Check sheet for the modelled part. Datum: model origin and axes. Units: mm. A direction names the side the tool comes from. Coordinates: 2 decimals unless noted, no trailing zeros. Loops run counter-clockwise (first coordinate to the right, second up) from the corner with the lowest first, then second, coordinate; pieces in that order, holes last. Notation, with made-up numbers: (84.5, 74) - (127.5, 74) arc R26 cw to (127.5, 91) - close; hole circle Ø11 at (3.25, -8.5). An arc over 180 degrees is marked (long way). Write each question's results on one line, items separated by ' | '. Start each with the question number.
1. Cross-section at C-C (y = -9). Record the cut outline in (x, z).
2. Thickness scan on line 1 (X direction, y = -5.5, z = 2.25); line 2 (X direction, y = 11, z = 1.5); line 3 (X direction, y = -10.5, z = 2). Record the ranges inside material, lowest first. Write a range as [from, to].
3. Draft check along X on faces 5 (the face through (40.14, 0.28, 5.9)), 6 (the face through (43, 0, 17)), 7 (the face through (17.5, -13, 2)). Enter one of: released by +X, released by -X, zero draft, split by the parting line, or undercut.
4. Gauge pin test, flat ends, axial feed: P1, Ø2.5, axis at y = -15.5, z = 3, coming from the -X side; P2, Ø2.5, axis at y = 5.5, z = 13, coming from the -X side; P3, Ø1.5, axis at x = -16, z = 3, coming from the -Y side; P4, Ø1.5, axis at y = 13.5, z = 1.5, coming from the -X side. Record the tip position at first contact, or that the pin passes through.
5. Cross-section at D-D (y = -16). Record the cut outline in (x, z), and give its area (3 significant figures).
6. Cross-section at A-A (z = 12). Record the cut outline in (x, y), and give its area (3 significant figures).
7. Cross-section at B-B (y = 4). Record the cut outline in (x, z), and give its area (3 significant figures).
8. Tool access check on faces 1 (the face through (27, -5.91, 2)), 2 (the face through (36, 15, 2)), 3 (the face through (43.465, 13.376, 12.066)), 4 (the face through (41, 0, 12)). Record the directions out of +Z, -Z, +X, -X, +Y, -Y that give a thin tool (end or side, any length) a straight path to the whole face; none if there is none.
```python
from build123d import *

# Parameters (mm, degrees)
F1_DEPTH = 5
F2_W     = 5
F2_H     = 40
F3_DEPTH = 12
F4_R     = 3
F5_R     = 1.5
F6_DEPTH = 10


with BuildPart() as f1:
    # F0 (on Top) → F1 (new body)
    with BuildSketch(Plane.XY):
        with BuildLine():
            Line((36, 18), (36, 10.910335))
            ThreePointArc((36, 10.910335), (34.535534, 7.374801), (31, 5.910335))
            Line((31, 5.910335), (19.677769, 5.910335))
            ThreePointArc((19.677769, 5.910335), (17.140309, 6.602052), (15.304931, 8.485816))
            ThreePointArc((15.304931, 8.485816), (-4.382562, 16.942348), (-17.5, 0))
            Line((-17.5, 0), (-17.5, -15))
            Line((-17.5, -15), (-12, -15))
            Line((-12, -15), (-12, 0))
            ThreePointArc((-12, 0), (0, 12), (12, 0))
            Line((12, 0), (12, -15))
            Line((12, -15), (17.5, -15))
            Line((17.5, -15), (17.5, -10.910335))
            ThreePointArc((17.5, -10.910335), (18.964466, -7.374801), (22.5, -5.910335))
            Line((22.5, -5.910335), (31, -5.910335))
            ThreePointArc((31, -5.910335), (34.535534, -7.374801), (36, -10.910335))
            Line((36, -10.910335), (36, -18))
            ThreePointArc((36, -18), (36.585786, -19.414214), (38, -20))
            Line((38, -20), (46, -20))
            Line((46, -20), (46, 0))
            Line((46, 0), (46, 20))
            Line((46, 20), (38, 20))
            ThreePointArc((38, 20), (36.585786, 19.414214), (36, 18))
        make_face()
    extrude(amount=F1_DEPTH)

    # F2 (on face) → F3 (join)
    with BuildSketch(Plane.XY.offset(5)):
        with Locations((43.5, 0)):
            Rectangle(F2_W, F2_H)
    extrude(amount=F3_DEPTH)

    # F4
    f4_edges = [f1.edges().sort_by_distance(p)[0] for p in [
        (41, 0, 5),
        (43.5, 20, 17),
        (43.5, -20, 17),
    ]]
    fillet(f4_edges, radius=F4_R)

    # F5 (on face) → F6 (cut)
    with BuildSketch(Plane(origin=(41, 0, 0), x_dir=(0, -1, 0), z_dir=(-1, 0, 0))):
        with Locations((-11.877556, 12)):
            Circle(F5_R)
        with Locations((11.877556, 12)):
            Circle(F5_R)
    extrude(amount=-F6_DEPTH, mode=Mode.SUBTRACT)


solid = f1.part
```
Established:
1) outline: (-17.5, 0) - (-12, 0) - (-12, 5) - (-17.5, 5) - close; (12, 0) - (17.88, 0) - (17.88, 5) - (12, 5) - close; (35.62, 0) - (46, 0) - (46, 17) - (41, 17) - (41, 8) arc R3 cw to (38, 5) - (35.62, 5) - close
2) line 1: [-17.5, -12], [12, 46] | line 2: [-13.61, -4.8], [4.8, 13.61], [36, 46] | line 3: [-17.5, -12], [12, 17.52], [35.98, 46]
3) face 5: released by -X | face 6: zero draft | face 7: undercut
4) P1: x = -17.5 | P2: x = 41 | P3: y = -15 | P4: x = -11.99
5) outline: (36, 0) - (46, 0) - (46, 17) - (41, 17) - (41, 8) arc R3 cw to (38, 5) - (36, 5) - close | area: 112 mm^2
6) outline: (41, -20) - (46, -20) - (46, -13.38) - (41, -13.38) - close; (41, -10.38) - (46, -10.38) - (46, 10.38) - (41, 10.38) - close; (41, 13.38) - (46, 13.38) - (46, 20) - (41, 20) - close | area: 170 mm^2
7) outline: (-17.04, 0) - (-11.31, 0) - (-11.31, 5) - (-17.04, 5) - close; (11.31, 0) - (46, 0) - (46, 17) - (41, 17) - (41, 8) arc R3 cw to (38, 5) - (11.31, 5) - close | area: 264 mm^2
8) face 1: +Z, -Z, -Y | face 2: +Z, -Z, +Y | face 3: +X, -X | face 4: +Z, -X, +Y, -Y
